Part model, mm, in its own coordinate system. Give positions to 0.01 mm unless a question says otherwise; leave off trailing zeros. Order: outer loops, then holes, each group sorted by start corner. A loop starts at its lowest first (then second) coordinate and runs counter-clockwise, first axis right, second up.
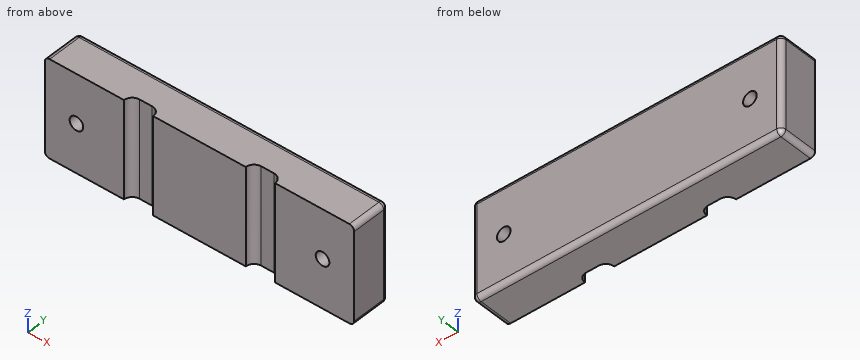
from build123d import *

# Parameters (mm, degrees)
SKETCH1_W            = 63.5
SKETCH1_H            = 20
SKETCH1_R            = 1.4
BASE_DEPTH           = 8
WIRE_GROOVES_DEPTH   = 39.833780398
F_1MM_EDGE_FILLETS_R = 1


with BuildPart() as part:
    # Sketch1 → Base (new body)
    with BuildSketch(Plane(origin=(0, 0, 0), x_dir=(1, 0, 0), z_dir=(0, 1, 0))):
        Rectangle(SKETCH1_W, SKETCH1_H)
        with Locations(Location((-25.25, 0, 0), (0, 0, 270))):
            Circle(SKETCH1_R, mode=Mode.SUBTRACT)
        with Locations(Location((25.25, 0, 0), (0, 0, 90))):
            Circle(SKETCH1_R, mode=Mode.SUBTRACT)
    extrude(amount=BASE_DEPTH)

    # Sketch2 → Wire Grooves (cut, through all)
    with BuildSketch(Plane(origin=(0, 10, -10), x_dir=(1, 0, 0), z_dir=(0, 0, -1))):
        with BuildLine():
            Line((-15.5, 10), (-9.5, 10))
            ThreePointArc((-9.5, 10), (-9.997918472, 8.797918472), (-11.2, 8.3))
            Line((-11.2, 8.3), (-13.8, 8.3))
            ThreePointArc((-13.8, 8.3), (-15.002081528, 8.797918472), (-15.5, 10))
        make_face()
        with BuildLine():
            Line((9.5, 10), (15.5, 10))
            ThreePointArc((15.5, 10), (15.002081528, 8.797918472), (13.8, 8.3))
            Line((13.8, 8.3), (11.2, 8.3))
            ThreePointArc((11.2, 8.3), (9.997918472, 8.797918472), (9.5, 10))
        make_face()
    extrude(amount=-WIRE_GROOVES_DEPTH, mode=Mode.SUBTRACT)

    # 1mm Edge Fillets
    f_1mm_edge_fillets_edges = [part.edges().sort_by_distance(p)[0] for p in [
        (31.75, 8, 0),
        (0, 8, -10),
        (-31.75, 8, 0),
        (-31.75, 4, -10),
        (31.75, 4, -10),
        (31.75, 4, 10),
        (-31.75, 4, 10),
        (0, 8, 10),
    ]]
    fillet(f_1mm_edge_fillets_edges, radius=F_1MM_EDGE_FILLETS_R)


solid = part.part
Item 1: Band-saw the part on D-D on x = -13. List the corners of the cut face in (y, z), plus the area to 3 significant figures.
Item 2: Band-saw the part on A-A on z = 0. List the corners of the cut face in (x, y).
Item 3: Drill centre lines: probe 1 along X at (y, z) = (1, 7); probe 2 along X at (y, z) = (1.5, 5.5); probe 3 along X at (y, z) = (1.5, 0). Where is each one in solid material? Low to high.
Item 4: Band-saw the part on B-B on x = -25.25. List the corners of the cut face in (y, z), plus the area to 3 significant figures.
Item 5: Drop flat-ended pins along their axis: P1, Ø5, axis at x = -5.5, z = 3, coming from the -Y side; P2, Ø0.8, axis at x = 13, z = -3, coming from the -Y side. Give the stop position or say it passes through.
Item 6: Band-saw the part on C-C on z = 6.5. List the corners of the cut face in (x, y), plus the area to 3 significant figures.
Working result:
1. outline: (1.7, -10) - (7, -10) arc R1 ccw to (8, -9) - (8, 9) arc R1 ccw to (7, 10) - (1.7, 10) - close
1. area: 126 mm2
2. outline: (-31.75, 0) - (-26.65, 0) - (-26.65, 8) - (-30.75, 8) arc R1 ccw to (-31.75, 7) - close; (-23.85, 0) - (-15.5, 0) arc R1.7 cw to (-13.8, 1.7) - (-11.2, 1.7) arc R1.7 cw to (-9.5, 0) - (9.5, 0) arc R1.7 cw to (11.2, 1.7) - (13.8, 1.7) arc R1.7 cw to (15.5, 0) - (23.85, 0) - (23.85, 8) - (-23.85, 8) - close; (26.65, 0) - (31.75, 0) - (31.75, 7) arc R1 ccw to (30.75, 8) - (26.65, 8) - close
3. probe 1: x = -31.75 to -15.17, -9.83 to 9.83, 15.17 to 31.75
3. probe 2: x = -31.75 to -14.6, -10.4 to 10.4, 14.6 to 31.75
3. probe 3: x = -31.75 to -26.65, -23.85 to -14.6, -10.4 to 10.4, 14.6 to 23.85, 26.65 to 31.75
4. outline: (0, -10) - (7, -10) arc R1 ccw to (8, -9) - (8, -1.4) - (0, -1.4) - close; (0, 1.4) - (8, 1.4) - (8, 9) arc R1 ccw to (7, 10) - (0, 10) - close
4. area: 137 mm2
5. P1: stops at y = 0
5. P2: stops at y = 1.7
6. outline: (-31.75, 0) - (-15.5, 0) arc R1.7 cw to (-13.8, 1.7) - (-11.2, 1.7) arc R1.7 cw to (-9.5, 0) - (9.5, 0) arc R1.7 cw to (11.2, 1.7) - (13.8, 1.7) arc R1.7 cw to (15.5, 0) - (31.75, 0) - (31.75, 7) arc R1 ccw to (30.75, 8) - (-30.75, 8) arc R1 ccw to (-31.75, 7) - close
6. area: 490 mm2
